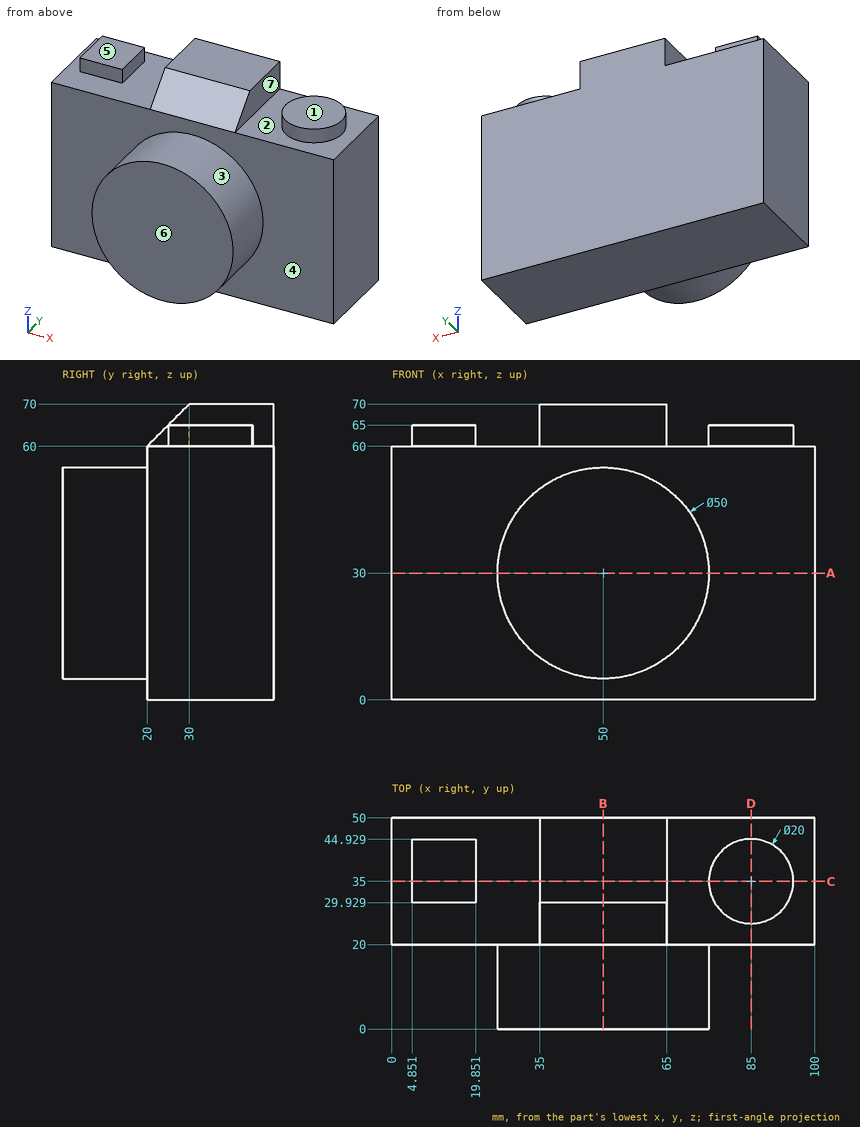
The figure shows three views and two pictorial views of one solid part (mm, origin at its lowest corner). Answer the questions. A direction names the side the tool comes from. Give positions to 0.01 mm unless a question says otherwise; leave off trailing zeros. Order: outer loops, then holes, each group sorted by start corner. A loop starts at its lowest first (then second) coordinate and runs counter-clockwise, first axis right, second up. Notation, with made-up numbers: (77.25, 46.5) -> (87.25, 46.5) arc R17 cw to (87.25, 56.5) -> close; hole circle Ø7 at (-12, 40.5). An arc over 180 degrees is marked (long way). Answer as a JSON object with one key per item and string values. Group by question number.
Item 1: Determine the mould class of the marked faces 1, 2 and 3 for opening direction X: pulls with the +X half, pulls with the -X half, needs draft (parallel to the pull), parting line crosses it, or undercut.
Item 2: A tool of negligible diameter and unlimited length cuts with its end or side. For the marked faces 4, 5, 6 and 7, from which of +Z, -Z, +X, -X, +Y, -Y can it reach the whole face along a straight path? Write none if from no direction.
Item 3: The part is cut by section C-C on y = 35. Write down the section's boundary in (x, z), and give its area (4 significant figures).
Item 4: The part is cut by section D-D on x = 85. Write down the section's boundary in (y, z), and give its area (3 significant figures).
Item 5: Flat-ended cylindrical pins translate along their axes: pin 1 (1 mm diameter, centred on x = 82, y = 43.5, fed in from +Z); pin 2 (3 mm diameter, centred on y = 34.5, z = 65.5, fed in from +X); pin 3 (3 mm diameter, centred on y = 37.5, z = 14.5, fed in from -X); pin 4 (4 mm diameter, centred on y = 39, z = 62.5, fed in from +X). Find the tip coordinate at first contact, or state that the pin passes through.
Item 6: The part is cut by section B-B on x = 50. Write down the section's boundary in (y, z).
Item 7: The part is cut by section A-A on z = 30. Write down the section's boundary in (x, y), and give its area (3 significant figures).
Item 8: Consider L1, parallel to X at y = 37, z = 61; L2, parallel to Y at x = 40.5, z = 55.5; L3, parallel to Y at x = 16.5, z = 64. Determine where each line is inside the solid, lowest interval first. Write a range as from..to.
Result set:
{
 "1": {"face 1": "needs draft", "face 2": "undercut", "face 3": "parting line crosses it"},
 "2": {"face 4": "-Y", "face 5": "+Z, -X, +Y, -Y", "face 6": "+Z, -Z, +X, -X, -Y", "face 7": "+Z, +Y, -Y"},
 "3": {"outline": "(0, 0) -> (100, 0) -> (100, 60) -> (95, 60) -> (95, 65) -> (75, 65) -> (75, 60) -> (65, 60) -> (65, 70) -> (35, 70) -> (35, 60) -> (19.85, 60) -> (19.85, 65) -> (4.85, 65) -> (4.85, 60) -> (0, 60) -> close", "area": "6,475 mm²"},
 "4": {"outline": "(20, 0) -> (50, 0) -> (50, 60) -> (45, 60) -> (45, 65) -> (25, 65) -> (25, 60) -> (20, 60) -> close", "area": "1,900 mm²"},
 "5": {"pin 1": "z = 65", "pin 2": "x = 95", "pin 3": "x = 0", "pin 4": "x = 94.8"},
 "6": {"outline": "(0, 5) -> (20, 5) -> (20, 0) -> (50, 0) -> (50, 70) -> (30, 70) -> (20, 60) -> (20, 55) -> (0, 55) -> close"},
 "7": {"outline": "(0, 20) -> (25, 20) -> (25, 0) -> (75, 0) -> (75, 20) -> (100, 20) -> (100, 50) -> (0, 50) -> close", "area": "4,000 mm²"},
 "8": {"L1": "4.85..19.85, 35..65, 75.2..94.8", "L2": "20..50", "L3": "29.93..44.93"}
}
